Read the model definition and answer for the solid it produces. Units are mm, in the model's axes. Face numbers are marked on the shaded views. A direction names the side the tool comes from. Coordinates: 2 decimals unless noted, no trailing zeros. Write each loop counter-clockwise with the first axis right and the second up, starting at its lowest first coordinate (ties: lowest second). Pieces come first, ordered by that corner, then holes.
(1) The part is cut by section A-A, the plane z = 54. State how many separate pieces and enclosed holes the cut face has, and give its area (3 significant figures).
(2) The part is cut by section B-B, the plane y = 10. Determine the outline of the cut face in (x, z) (1 decimal), and give its area (3 significant figures).
(3) The part is cut by section C-C, the plane x = 158. Determine the outline of the cut face in (y, z) (3 decimals), and give its area (3 significant figures).
(4) Straight lines are drawn through the part: line 1 along X through (y, z) = (-95, 189.5); line 2 along Y through (x, z) = (50, 41.5); line 3 along X through (y, z) = (-164.5, 141). For each, find the intervals that lie inside material, in ascending order.
(5) The part is cut by section D-D, the plane y = -176. Determine the outline of the cut face in (x, z) (1 decimal), and give its area (3 significant figures).
(6) Determine the mould class of the marked faces 1, 2, 3 and 4 for opening direction X: pulls with the +X half, pulls with the -X half, needs draft (parallel to the pull), parting line crosses it, or undercut.
(7) Which of the six approach directions +Z, -Z, +X, -X, +Y, -Y give full straight-line access (tool end or side, diameter ignored) to the marked faces 5, 6 and 7?
(8) Given pin 1 (1 mm diameter, centred on x = -2, z = 195.5, fed in from -Y); pin 2 (1.5 mm diameter, centred on x = -149, y = -64, fed in from +Z) (3 decimals); pin 3 (12 mm diameter, centred on x = -169.5, z = 57, fed in from -Y), each flat-ended and moving along its own axis, determine where each tip first touches the part or whether it passes through.
```python
from build123d import *

# Parameters (mm, degrees)
SKETCH1_W           = 558.803
SKETCH1_H           = 314.432
SKETCH1_W_2         = 552.453
SKETCH1_H_2         = 308.082
SKETCH1_W_3         = 3.175
SKETCH1_W_4         = 89.789
SKETCH1_W_5         = 87.632
SKETCH1_W_6         = 89.79
SKETCH1_H_3         = 57.15
BOSS_EXTRUDE1_DEPTH = 3.175
SKETCH2_W           = 558.803
SKETCH2_H           = 371.582
SKETCH2_W_2         = 89.79
SKETCH2_H_2         = 308.082
SKETCH2_W_3         = 89.789
SKETCH2_W_4         = 552.453
SKETCH2_H_3         = 53.975
SKETCH2_W_5         = 87.632
BOSS_EXTRUDE2_DEPTH = 176.6
SKETCH4_W           = 552.453
SKETCH4_H           = 176.6
CUT_EXTRUDE1_DEPTH  = 3.175
SKETCH5_W           = 87.632
SKETCH5_H           = 308.082
SKETCH5_W_2         = 89.789
SKETCH5_W_3         = 89.79
BOSS_EXTRUDE5_DEPTH = 38.1
SKETCH7_W           = 3.175
SKETCH7_H           = 308.082
CUT_EXTRUDE2_DEPTH  = 35


with BuildPart() as part:
    # Sketch1 → Boss-Extrude1 (new body)
    # profile 1 of 13: a face of its own
    with BuildSketch(Plane.XY):
        Rectangle(SKETCH1_W, SKETCH1_H)
        Rectangle(SKETCH1_W_2, SKETCH1_H_2, mode=Mode.SUBTRACT)
    # profile 2 of 13: a face of its own
    with BuildSketch(Plane.XY):
        with Locations((-187.007, 0)):
            Rectangle(SKETCH1_W_3, SKETCH1_H_2)
    # profile 3 of 13: a face of its own
    with BuildSketch(Plane.XY):
        with Locations((-140.525, 0)):
            Rectangle(SKETCH1_W_4, SKETCH1_H_2)
    # profile 4 of 13: a face of its own
    with BuildSketch(Plane.XY):
        with Locations((-232.4105, 0)):
            Rectangle(SKETCH1_W_5, SKETCH1_H_2)
    # profile 5 of 13: a face of its own
    with BuildSketch(Plane.XY):
        with Locations((-47.561, 0)):
            Rectangle(SKETCH1_W_4, SKETCH1_H_2)
    # profile 6 of 13: a face of its own
    with BuildSketch(Plane.XY):
        with Locations((-94.043, 0)):
            Rectangle(SKETCH1_W_3, SKETCH1_H_2)
    # profile 7 of 13: a face of its own
    with BuildSketch(Plane.XY):
        with Locations((45.403, 0)):
            Rectangle(SKETCH1_W_4, SKETCH1_H_2)
    # profile 8 of 13: a face of its own
    with BuildSketch(Plane.XY):
        with Locations((-1.079, 0)):
            Rectangle(SKETCH1_W_3, SKETCH1_H_2)
    # profile 9 of 13: a face of its own
    with BuildSketch(Plane.XY):
        with Locations((138.367, 0)):
            Rectangle(SKETCH1_W_4, SKETCH1_H_2)
    # profile 10 of 13: a face of its own
    with BuildSketch(Plane.XY):
        with Locations((91.885, 0)):
            Rectangle(SKETCH1_W_3, SKETCH1_H_2)
    # profile 11 of 13: a face of its own
    with BuildSketch(Plane.XY):
        with Locations((231.3315, 0)):
            Rectangle(SKETCH1_W_6, SKETCH1_H_2)
    # profile 12 of 13: a face of its own
    with BuildSketch(Plane.XY):
        with Locations((184.849, 0)):
            Rectangle(SKETCH1_W_3, SKETCH1_H_2)
    # profile 13 of 13: a face of its own
    with BuildSketch(Plane.XY):
        with Locations((0, -185.791)):
            Rectangle(SKETCH1_W, SKETCH1_H_3)
    extrude(amount=BOSS_EXTRUDE1_DEPTH)

    # Sketch2 → Boss-Extrude2 (add)
    with BuildSketch(Plane.XY.offset(3.175)):
        with Locations((0, -28.575)):
            Rectangle(SKETCH2_W, SKETCH2_H)
        with Locations((231.3315, 0)):
            Rectangle(SKETCH2_W_2, SKETCH2_H_2, mode=Mode.SUBTRACT)
        with Locations((138.367, 0)):
            Rectangle(SKETCH2_W_3, SKETCH2_H_2, mode=Mode.SUBTRACT)
        with Locations((0, -184.2035)):
            Rectangle(SKETCH2_W_4, SKETCH2_H_3, mode=Mode.SUBTRACT)
        with Locations((45.403, 0)):
            Rectangle(SKETCH2_W_3, SKETCH2_H_2, mode=Mode.SUBTRACT)
        with Locations((-47.561, 0)):
            Rectangle(SKETCH2_W_3, SKETCH2_H_2, mode=Mode.SUBTRACT)
        with Locations((-140.525, 0)):
            Rectangle(SKETCH2_W_3, SKETCH2_H_2, mode=Mode.SUBTRACT)
        with Locations((-232.4105, 0)):
            Rectangle(SKETCH2_W_5, SKETCH2_H_2, mode=Mode.SUBTRACT)
    extrude(amount=BOSS_EXTRUDE2_DEPTH)

    # Sketch4 → Cut-Extrude1 (cut)
    with BuildSketch(Plane.XZ.offset(214.366)):
        with Locations((0, 91.475)):
            Rectangle(SKETCH4_W, SKETCH4_H)
    extrude(amount=-CUT_EXTRUDE1_DEPTH, mode=Mode.SUBTRACT)

    # Sketch5 → Boss-Extrude5 (add)
    with BuildSketch(Plane.XY.offset(179.775)):
        Polygon((-279.4015, 157.216), (-279.4015, -214.366), (-276.2265, -214.366), (-276.2265, -157.216), (276.2265, -157.216), (276.2265, -214.366), (279.4015, -214.366), (279.4015, 157.216), align=None)
        with Locations((-232.4105, 0)):
            Rectangle(SKETCH5_W, SKETCH5_H, mode=Mode.SUBTRACT)
        with Locations((-140.525, 0)):
            Rectangle(SKETCH5_W_2, SKETCH5_H, mode=Mode.SUBTRACT)
        with Locations((-47.561, 0)):
            Rectangle(SKETCH5_W_2, SKETCH5_H, mode=Mode.SUBTRACT)
        with Locations((45.403, 0)):
            Rectangle(SKETCH5_W_2, SKETCH5_H, mode=Mode.SUBTRACT)
        with Locations((138.367, 0)):
            Rectangle(SKETCH5_W_2, SKETCH5_H, mode=Mode.SUBTRACT)
        with Locations((231.3315, 0)):
            Rectangle(SKETCH5_W_3, SKETCH5_H, mode=Mode.SUBTRACT)
    extrude(amount=BOSS_EXTRUDE5_DEPTH)

    # Sketch7 → Cut-Extrude2 (cut)
    with BuildSketch(Plane.XY.offset(217.875)):
        Polygon((-185.4195, -154.041), (-188.5945, -154.041), (-276.2265, -154.041), (-276.2265, -157.216), (276.2265, -157.216), (276.2265, -154.041), (186.4365, -154.041), (183.2615, -154.041), (93.4725, -154.041), (90.2975, -154.041), (0.5085, -154.041), (-2.6665, -154.041), (-92.4555, -154.041), (-95.6305, -154.041), align=None)
        with Locations((184.849, 0)):
            Rectangle(SKETCH7_W, SKETCH7_H)
    extrude(amount=-CUT_EXTRUDE2_DEPTH, mode=Mode.SUBTRACT)


solid = part.part
```
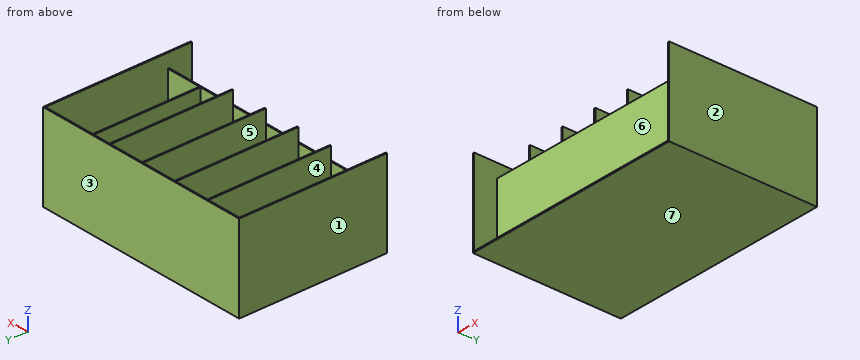
Computed:
1. separate pieces: 1
1. enclosed holes: 6
1. area: 10,800 mm2
2. outline: (-279.4, 0) - (279.4, 0) - (279.4, 217.9) - (276.2, 217.9) - (276.2, 3.2) - (186.4, 3.2) - (186.4, 182.9) - (183.3, 182.9) - (183.3, 3.2) - (93.5, 3.2) - (93.5, 217.9) - (90.3, 217.9) - (90.3, 3.2) - (0.5, 3.2) - (0.5, 217.9) - (-2.7, 217.9) - (-2.7, 3.2) - (-92.5, 3.2) - (-92.5, 217.9) - (-95.6, 217.9) - (-95.6, 3.2) - (-185.4, 3.2) - (-185.4, 217.9) - (-188.6, 217.9) - (-188.6, 3.2) - (-276.2, 3.2) - (-276.2, 217.9) - (-279.4, 217.9) - close
2. area: 6,430 mm2
3. outline: (-214.366, 0) - (157.216, 0) - (157.216, 217.875) - (154.041, 217.875) - (154.041, 3.175) - (-154.041, 3.175) - (-154.041, 182.875) - (-157.216, 182.875) - (-157.216, 3.175) - (-214.366, 3.175) - close
3. area: 2,430 mm2
4. line 1: x = -279.4 to -276.23, -188.59 to -185.42, -95.63 to -92.46, -2.67 to 0.51, 90.3 to 93.47, 276.23 to 279.4
4. line 2: y = -157.22 to -154.04, 154.04 to 157.22
4. line 3: x = -279.4 to -276.23, 276.23 to 279.4
5. outline: (-279.4, 0) - (279.4, 0) - (279.4, 217.9) - (276.2, 217.9) - (276.2, 3.2) - (-276.2, 3.2) - (-276.2, 217.9) - (-279.4, 217.9) - close
5. area: 3,140 mm2
6. face 1: pulls with the -X half
6. face 2: pulls with the +X half
6. face 3: needs draft
6. face 4: undercut
7. face 5: +Z
7. face 6: +Z, -Y
7. face 7: -Z, +X, -X, +Y, -Y
8. pin 1: stops at y = -154.04
8. pin 2: stops at z = 3.175
8. pin 3: stops at y = -157.22
